from build123d import *

# Parameters (mm, degrees)
SCHIZZO13_R                  = 1.25
SCHIZZO13_R_2                = 1.5
SCHIZZO13_R_3                = 2.75
ESTRUSIONE_ESTRUSIONE2_DEPTH = 6


with BuildPart() as part:
    # Schizzo13 → Estrusione-Estrusione2 (new body)
    with BuildSketch(Plane.XY):
        with BuildLine():
            Line((10, 0), (24.28195797, 0))
            Line((24.28195797, 0), (34.28195797, 10))
            Line((34.28195797, 10), (34.28195797, 30))
            Line((34.28195797, 30), (57.017366293, 53.192694567))
            Line((57.017366293, 53.192694567), (83.745372993, 53.192694567))
            Line((83.745372993, 53.192694567), (107.404551383, 30))
            Line((107.404551383, 30), (107.404551383, 10))
            Line((107.404551383, 10), (117.404551383, 0))
            Line((117.404551383, 0), (232.595448617, 0))
            Line((232.595448617, 0), (242.595448617, 10))
            Line((242.595448617, 10), (242.595448617, 30))
            Line((242.595448617, 30), (266.254627007, 53.192694567))
            Line((266.254627007, 53.192694567), (292.982633707, 53.192694567))
            Line((292.982633707, 53.192694567), (315.71804203, 30))
            Line((315.71804203, 30), (315.71804203, 10))
            Line((315.71804203, 10), (325.71804203, 0))
            Line((325.71804203, 0), (340, 0))
            Line((340, 0), (350, 10))
            Line((350, 10), (350, 70.5))
            Line((350, 70.5), (292.919241786, 124.388863529))
            Line((292.919241786, 124.388863529), (292.919241786, 225.611136471))
            Line((292.919241786, 225.611136471), (350, 279.5))
            Line((350, 279.5), (350, 340))
            Line((350, 340), (340, 350))
            Line((340, 350), (302.982633707, 350))
            Line((302.982633707, 350), (292.982633707, 340))
            Line((292.982633707, 340), (292.982633707, 299.807305433))
            ThreePointArc((292.982633707, 299.807305433), (292.103954051, 297.685985089), (289.982633707, 296.807305433))
            Line((289.982633707, 296.807305433), (266.254627007, 296.807305433))
            Line((266.254627007, 296.807305433), (242.595448617, 320))
            Line((242.595448617, 320), (242.595448617, 340))
            Line((242.595448617, 340), (232.595448617, 350))
            Line((232.595448617, 350), (188.89112909, 350))
            Line((188.89112909, 350), (182.89112909, 344))
            Line((182.89112909, 344), (167.10887091, 344))
            Line((167.10887091, 344), (161.10887091, 350))
            Line((161.10887091, 350), (117.404551383, 350))
            Line((117.404551383, 350), (107.404551383, 340))
            Line((107.404551383, 340), (107.404551383, 320))
            Line((107.404551383, 320), (83.745372993, 296.807305433))
            Line((83.745372993, 296.807305433), (57.017366293, 296.807305433))
            Line((57.017366293, 296.807305433), (34.28195797, 320))
            Line((34.28195797, 320), (34.28195797, 340))
            Line((34.28195797, 340), (24.28195797, 350))
            Line((24.28195797, 350), (10, 350))
            Line((10, 350), (0, 340))
            Line((0, 340), (0, 279.5))
            Line((0, 279.5), (57.080758214, 225.611136471))
            Line((57.080758214, 225.611136471), (57.080758214, 175))
            Line((57.080758214, 175), (57.080758214, 124.388863529))
            Line((57.080758214, 124.388863529), (0, 70.5))
            Line((0, 70.5), (0, 10))
            Line((0, 10), (10, 0))
        make_face()
        with Locations((15, 320)):
            Circle(SCHIZZO13_R, mode=Mode.SUBTRACT)
        with Locations((20.5, 279.5)):
            Circle(SCHIZZO13_R, mode=Mode.SUBTRACT)
        with Locations((57.080758214, 279.5)):
            Circle(SCHIZZO13_R, mode=Mode.SUBTRACT)
        with Locations((175, 175)):
            Circle(SCHIZZO13_R_2, mode=Mode.SUBTRACT)
        with Locations((20.5, 70.5)):
            Circle(SCHIZZO13_R, mode=Mode.SUBTRACT)
        with Locations((200, 344)):
            Circle(SCHIZZO13_R_3, mode=Mode.SUBTRACT)
        with Locations((150, 344)):
            Circle(SCHIZZO13_R_3, mode=Mode.SUBTRACT)
        with Locations((175, 329)):
            Circle(SCHIZZO13_R_3, mode=Mode.SUBTRACT)
        with Locations((217, 329)):
            Circle(SCHIZZO13_R_3, mode=Mode.SUBTRACT)
        with Locations((133, 329)):
            Circle(SCHIZZO13_R_3, mode=Mode.SUBTRACT)
        with Locations((70.5, 70.5)):
            Circle(SCHIZZO13_R, mode=Mode.SUBTRACT)
        with Locations((279.5, 70.5)):
            Circle(SCHIZZO13_R, mode=Mode.SUBTRACT)
        with Locations((329.5, 70.5)):
            Circle(SCHIZZO13_R, mode=Mode.SUBTRACT)
        with Locations((335, 10)):
            Circle(SCHIZZO13_R, mode=Mode.SUBTRACT)
        with Locations((15, 10)):
            Circle(SCHIZZO13_R, mode=Mode.SUBTRACT)
        with Locations((279.5, 279.5)):
            Circle(SCHIZZO13_R, mode=Mode.SUBTRACT)
        with Locations((329.5, 279.5)):
            Circle(SCHIZZO13_R, mode=Mode.SUBTRACT)
        with Locations((335, 320)):
            Circle(SCHIZZO13_R, mode=Mode.SUBTRACT)
        with Locations((310, 344)):
            Circle(SCHIZZO13_R, mode=Mode.SUBTRACT)
        with Locations((330, 344)):
            Circle(SCHIZZO13_R, mode=Mode.SUBTRACT)
        Polygon((217, 193.286910978), (227.343033378, 225.611136471), (185.750894453, 266.383210572), (164.249105547, 266.383210572), (122.656966622, 225.611136471), (133, 193.286910978), align=None, mode=Mode.SUBTRACT)
        Polygon((133, 156.713089022), (101.348199345, 83.616789428), (155.254193112, 30), (194.745806888, 30), (248.651800655, 83.616789428), (217, 156.713089022), align=None, mode=Mode.SUBTRACT)
    extrude(amount=-ESTRUSIONE_ESTRUSIONE2_DEPTH)


solid = part.part
Input: part model. Units: mm. Frame: model coordinates. A direction names the side the tool comes from. Coordinates: 2 decimals unless noted, no trailing zeros. Loops run counter-clockwise (first coordinate to the right, second up) from the corner with the lowest first, then second, coordinate; pieces in that order, holes last.
(1) Material intervals for probe 1 along Y at (x, z) = (175, -3.35); probe 2 along X at (y, z) = (279.5, -1.7); probe 3 along X at (y, z) = (17.5, -4.8), sorted ascending.
(2) Section C-C on z = -2.65. Count the separate pieces of the cut face and the enclosed holes in it, then the cut area to 3 significant figures.
(3) Section A-A on x = 140.5. Return the cut outline in (y, z).
(4) Section D-D on y = 143. Return the cut outline in (x, z).
(5) First-contact query: pin 1 Ø2 at (x, y) = (70.5, 70.5) entering from -Z; pin 2 Ø1.8 at (x, z) = (283.5, -2) entering from -Y. Flat tips, straight axial feed; report the tip coordinate or a pass-through.
(6) Section B-B on y = 93. Return the cut outline in (x, z).
(7) Pull-direction query (Y, two-part tool) for faces 1 (the face through (127.924, 57.184, -2.958)), 2 (the face through (95.41, 41.76, -2.96)), 3 (the face through (5, 345, -3)); classes: released by +Y, released by -Y, zero draft, split by the parting line, or undercut.
(8) Set-up query: faces 4 (the face through (45.491, 41.434, -2.958)), 5 (the face through (112.475, 345.07, -2.958)), 6 (the face through (206.84, 245.71, -2.96)). Return all of +Z, -Z, +X, -X, +Y, -Y with unobstructed straight access to the full face (end or side cutting, diameter ignored); none if empty.
Data:
1. probe 1: y = 0 to 30, 156.71 to 173.5, 176.5 to 193.29, 266.38 to 326.25, 331.75 to 344
1. probe 2: x = 0 to 19.25, 21.75 to 55.83, 58.33 to 278.25, 280.75 to 328.25, 330.75 to 350
1. probe 3: x = 0 to 34.28, 107.4 to 242.6, 315.72 to 350
2. separate pieces: 1
2. enclosed holes: 22
2. area: 72,300 mm2
3. outline: (0, -6) - (44.68, -6) - (44.68, 0) - (0, 0) - close; (156.71, -6) - (193.29, -6) - (193.29, 0) - (156.71, 0) - close; (243.1, -6) - (350, -6) - (350, 0) - (243.1, 0) - close
4. outline: (57.08, -6) - (127.06, -6) - (127.06, 0) - (57.08, 0) - close; (222.94, -6) - (292.92, -6) - (292.92, 0) - (222.94, 0) - close
5. pin 1: passes through
5. pin 2: stops at y = 53.19
6. outline: (23.83, -6) - (105.41, -6) - (105.41, 0) - (23.83, 0) - close; (244.59, -6) - (326.17, -6) - (326.17, 0) - (244.59, 0) - close
7. face 1: undercut
7. face 2: released by -Y
7. face 3: released by +Y
8. face 4: +Z, -Z, -Y
8. face 5: +Z, -Z, +Y
8. face 6: +Z, -Z
